```python
from build123d import *

# Parameters (mm, degrees)
F0_R     = 150
F1_DEPTH = 30
F2_R     = 5


with BuildPart() as f1:
    # F0 (on Top) → F1 (new body)
    with BuildSketch(Plane.XY):
        Circle(F0_R)
        Polygon((-12.5, -35), (0, -35), (12.5, -35), (12.5, -95), (-12.5, -95), align=None, mode=Mode.SUBTRACT)
        Polygon((-35.355339, 14.142136), (-77.781746, 56.568542), (-60.104076, 74.246212), (-17.67767, 31.819805), align=None, mode=Mode.SUBTRACT)
        Polygon((56.568542, 77.781746), (74.246212, 60.104076), (31.819805, 17.67767), (14.142136, 35.355339), align=None, mode=Mode.SUBTRACT)
    extrude(amount=F1_DEPTH)

    # F2
    f2_edges = [f1.edges().sort_by_distance(p)[0] for p in [
        (-150, 0, 30),
    ]]
    fillet(f2_edges, radius=F2_R)


solid = f1.part
```
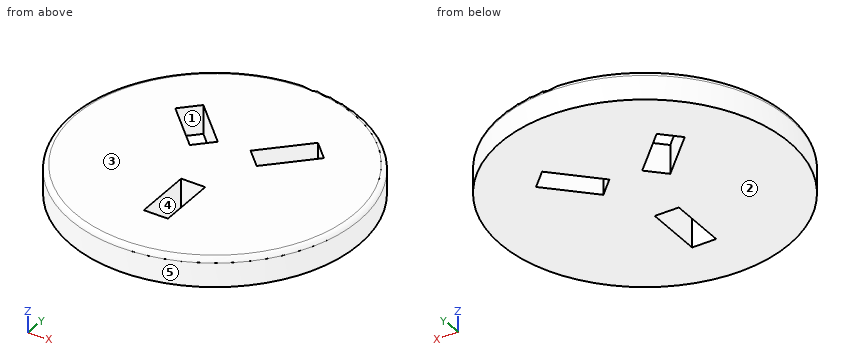
Can you work these out from the model? Positions are in its coordinate system, mm. Face numbers are marked on the shaded views. A direction names the side the tool comes from. Coordinates: 2 decimals unless noted, no trailing zeros. Write each loop counter-clockwise with the first axis right and the second up, starting at its lowest first coordinate (ties: lowest second). Pieces come first, ordered by that corner, then holes. Notation, with made-up numbers: M 83.5,61.5 L 142.5,61.5 A25 ccw 142.5,97.5 Z; hole C 46,48.25 d10. An arc over 180 degrees is marked long. Answer as CSV lines item,"result".
Item 1: Please list where these lines run through material, in increasing order: line 1 along X through (y, z) = (40.5, 11); line 2 along X through (y, z) = (34, 2.75); line 3 along Y through (x, z) = (-27.5, 8.75).
Geometry results:
line 1,"x = -144.43 to -61.71, -26.36 to 19.29, 54.64 to 144.43"
line 2,"x = -146.1 to -55.21, -19.86 to 15.5, 48.14 to 146.1"
line 3,"y = -147.46 to 22, 41.64 to 147.46"
Item 2: I'm going to push flat-ended pins straight in: P1, Ø12, axis at x = 75.5, z = 3, coming from the +Y side; P2, Ø12, axis at x = -13, z = 23, coming from the -Y side; P3, Ø1, axis at x = -26.5, z = 25, coming from the +Y side. Where does each tip first touch, or does it pass through?
Geometry results:
P1,"stops at y = 132.93"
P2,"stops at y = -149.84"
P3,"stops at y = 147.73"
Item 3: Imagine slicing it at B-B on x = 0. List the corners of the cut face in (y, z) for me, plus the area to 3 significant figures.
Geometry results:
outline,"M -150,0 L -95,0 L -95,30 L -145,30 A5 ccw -150,25 Z; M -35,0 L 150,0 L 150,25 A5 ccw 145,30 L -35,30 Z"
area,"7,190 mm2"
Item 4: We'd pull the mould along X, two halves only. Please class the marked faces 3, 4 and 5: +X half, -X half, draft (parallel to the pull), parting line (faces both ways), or undercut.
Geometry results:
face 3,"draft"
face 4,"undercut"
face 5,"parting line"
Item 5: On a 3-axis mill with a long thin cutter (end or side, diameter ignored), from which of +Z, -Z, +X, -X, +Y, -Y can I reach the whole of each face in a straight line? I mean the marked faces 1 and 2. Say none if no direction works.
Geometry results:
face 1,"+Z, -Z"
face 2,"-Z, +X, -X, +Y, -Y"
Item 6: Imagine slicing it at A-A on z = 17. List the corners of the cut face in (x, y) for me.
Geometry results:
outline,"C 0,0 d300; hole M -77.78,56.57 L -35.36,14.14 L -17.68,31.82 L -60.1,74.25 Z; hole M -12.5,-95 L 12.5,-95 L 12.5,-35 L -12.5,-35 Z; hole M 14.14,35.36 L 31.82,17.68 L 74.25,60.1 L 56.57,77.78 Z"
